Verification items for the finished model (mm, model axes). Face numbers are marked on the shaded views. A direction names the side the tool comes from. Give positions to 0.01 mm unless a question says otherwise; leave off trailing zeros. Order: outer loops, then holes, each group sorted by start corner. A loop starts at its lowest first (then second) coordinate and runs counter-clockwise, first axis right, second up. Notation, with made-up numbers: (76.5, -19.75) -> (117.5, -19.75) arc R12 cw to (117.5, -10.75) -> close; hole circle Ø9 at (6.5, 66.5). An arc over 180 degrees is marked (long way). Return JSON: item names as keys, results as strings. Group by question number.
(1) Release check for a two-part mould opening along Z. For the marked faces 3, 4, 5 and 6 record: pulls with the +Z half, pulls with the -Z half, needs draft (parallel to the pull), parting line crosses it, or undercut.
(2) Thickness scan on line 1 along X through (y, z) = (-2.75, -1.5); line 2 along Z through (x, y) = (-8.75, 1); line 3 along Y through (x, z) = (-10.5, 4.5). Record the ranges inside material, lowest first.
(3) Cross-section at C-C on x = -10.25. Enter the section's corners in (y, z).
(4) Cross-section at B-B on z = 3.5. Enter the section's corners in (x, y), then the cut area to 3 significant figures.
(5) Cross-section at A-A on y = -0.75. Enter the section's corners in (x, z), then the cut area to 3 significant figures.
(6) Cross-section at D-D on x = -6.25. Enter the section's corners in (y, z), then the cut area to 3 significant figures.
(7) Tool access check on the marked faces 1 and 2. Record the directions out of +Z, -Z, +X, -X, +Y, -Y that give a thin tool (end or side, any length) a straight path to the whole face; none if there is none.
(8) Depth check by flat-ended pin: pin 1 Ø1.5 at (y, z) = (1.5, 1) entering from +X; pin 2 Ø1.6 at (y, z) = (-2.5, -18.5) entering from +X; pin 3 Ø2 at (x, z) = (-14, 5.5) entering from +Y; pin 4 Ø2 at (y, z) = (2.5, 4.5) entering from -X. Enter the tip coordinate at first touch or a pass-through.
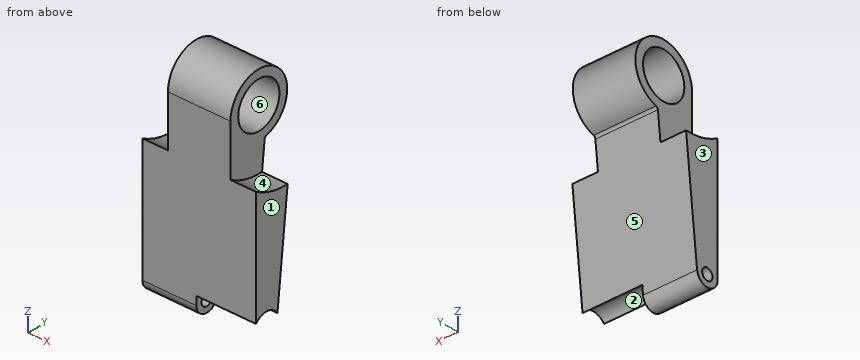
from build123d import *

# Parameters (mm, degrees)
SKETCH1_R           = 3.1369
SKETCH1_R_2         = 0.78486
BOSS_EXTRUDE1_DEPTH = 15.68196
FILLET1_R           = 0.39116
SKETCH2_R           = 8.23214
CUT_EXTRUDE1_DEPTH  = 3.52806
SKETCH3_R           = 8.23214
CUT_EXTRUDE2_DEPTH  = 3.52806
SKETCH4_R           = 1.96088
CUT_EXTRUDE3_DEPTH  = 8.23214


with BuildPart() as part:
    # Sketch1 → Boss-Extrude1 (new body)
    with BuildSketch(Plane(origin=(0, 0, 0), x_dir=(0, 0, -1), z_dir=(1, 0, 0))):
        with BuildLine():
            Line((-6.102081164, -4.312920003), (17.882851381, -4.312920003))
            ThreePointArc((17.882851381, -4.312920003), (19.449151228, -2.826510031), (18.046700375, -1.184608261))
            Line((18.046700375, -1.184608261), (-1.886270539, 0.910065763))
            ThreePointArc((-1.886270539, 0.910065763), (-9.458144317, 2.708896275), (-6.102081164, -4.312920003))
        make_face()
        with Locations((-6.102081164, -3e-09)):
            Circle(SKETCH1_R, mode=Mode.SUBTRACT)
        with Locations((17.882851381, -2.74447324)):
            Circle(SKETCH1_R_2, mode=Mode.SUBTRACT)
    extrude(amount=-BOSS_EXTRUDE1_DEPTH)

    # Fillet1
    fillet1_edges = [part.edges().sort_by_distance(p)[0] for p in [
        (-7.84098, 0.910065763, 1.886270539),
    ]]
    fillet(fillet1_edges, radius=FILLET1_R)

    # Sketch2 → Cut-Extrude1 (cut)
    with BuildSketch(Plane(origin=(0, 0, 0), x_dir=(0, 0, -1), z_dir=(1, 0, 0))):
        with Locations((-6.102081164, -3e-09)):
            Circle(SKETCH2_R)
    extrude(amount=-CUT_EXTRUDE1_DEPTH, mode=Mode.SUBTRACT)

    # Sketch3 → Cut-Extrude2 (cut)
    with BuildSketch(Plane.ZY.offset(15.68196)):
        with Locations((6.102081164, -3e-09)):
            Circle(SKETCH3_R)
    extrude(amount=-CUT_EXTRUDE2_DEPTH, mode=Mode.SUBTRACT)

    # Sketch4 → Cut-Extrude3 (cut)
    with BuildSketch(Plane(origin=(0, 0, 0), x_dir=(0, 0, -1), z_dir=(1, 0, 0))):
        with Locations((17.882851381, -2.74447324)):
            Circle(SKETCH4_R)
    extrude(amount=-CUT_EXTRUDE3_DEPTH, mode=Mode.SUBTRACT)


solid = part.part
Verdict:
{
 "1": {"face 3": "needs draft", "face 4": "pulls with the +Z half", "face 5": "pulls with the -Z half", "face 6": "undercut"},
 "2": {"line 1": "-12.15 to -3.53", "line 2": "1.86 to 3.13, 9.08 to 10.3", "line 3": "-4.31 to -2.7, 2.7 to 4"},
 "3": {"outline": "(-4.31, -17.88) arc R1.57 ccw to (-1.18, -18.05) -> (0.88, 1.61) arc R0.39 cw to (1.16, 1.95) arc R4.31 ccw (long way) to (-4.31, 6.1) -> close; hole circle Ø1.57 at (-2.74, -17.88); hole circle Ø6.27 at (0, 6.1)"},
 "4": {"outline": "(-12.15, -4.31) -> (-3.53, -4.31) -> (-3.53, -1.75) -> (-12.15, -1.75) -> close; (-12.15, 1.75) -> (-3.53, 1.75) -> (-3.53, 3.44) -> (-12.15, 3.44) -> close", "area": "36.6 mm²"},
 "5": {"outline": "(-15.68, -13.91) -> (0, -13.91) -> (0, -2.1) -> (-3.53, -2.1) -> (-3.53, 3.06) -> (-12.15, 3.06) -> (-12.15, -2.1) -> (-15.68, -2.1) -> close; (-12.15, 9.15) -> (-3.53, 9.15) -> (-3.53, 10.35) -> (-12.15, 10.35) -> close", "area": "240 mm²"},
 "6": {"outline": "(-4.31, -16.71) arc R1.96 cw to (-1.06, -16.88) -> (0.88, 1.61) arc R0.39 cw to (1.16, 1.95) arc R4.31 ccw (long way) to (-4.31, 6.1) -> close; hole circle Ø6.27 at (0, 6.1)", "area": "108 mm²"},
 "7": {"face 1": "+Z, -Z, +X, +Y, -Y", "face 2": "-Z, +X"},
 "8": {"pin 1": "x = -3.53", "pin 2": "x = -8.23", "pin 3": "through", "pin 4": "x = -12.15"}
}
